Build history of the part. All positions in model axes, mm. A direction names the side the tool comes from. Round coordinates to 2 decimals unless told otherwise and drop trailing zeros. Write each loop counter-clockwise with the first axis right and the second up, starting at its lowest first coordinate (ties: lowest second). Pieces come first, ordered by that corner, then holes. Notation, with made-up numbers: (34, 60.25) -> (80, 60.25) arc R27 cw to (80, 90.25) -> close; hole circle Ø9 at (77, 53.5). An arc over 180 degrees is marked (long way). Return JSON: item names as keys, results as strings.
from build123d import *

# Parameters (mm, degrees)
F0_R     = 6
F0_R_2   = 1.25
F3_DEPTH = 12
F4_DEPTH = 12


with BuildPart() as f2:
    # F2: sweep along a path in F1
    with BuildLine(Plane.XZ) as f2_path:
        Line((0, 0), (0, 5))
        ThreePointArc((0, 5), (4.3933982822, 15.6066017178), (15, 20))
        Line((15, 20), (54.5, 20))
        ThreePointArc((54.5, 20), (65.1066017178, 15.6066017178), (69.5, 5))
        Line((69.5, 5), (69.5, 0))
    # F0 (on Top) → F2 (sweep)
    with BuildSketch(Plane.XY):
        Circle(F0_R)
        Circle(F0_R_2, mode=Mode.SUBTRACT)
        Circle(F0_R_2)
    sweep(path=f2_path.line)

    # F0 (on Top) → F3 (cut)
    with BuildSketch(Plane.XY):
        Circle(F0_R_2)
    extrude(amount=F3_DEPTH, mode=Mode.SUBTRACT)

    # F0 (on Top) → F4 (cut)
    with BuildSketch(Plane.XY):
        with BuildLine():
            ThreePointArc((70.75, 0), (69.5, 1.25), (68.25, 0))
            ThreePointArc((68.25, 0), (69.5, -1.25), (70.75, 0))
        make_face()
    extrude(amount=F4_DEPTH, mode=Mode.SUBTRACT)


solid = f2.part
Q1. Wall check: L1, parallel to Y at x = 0, z = 8.5; L2, parallel to X at y = 0.5, z = 11.5; L3, parallel to X at y = 3.5, z = 3. Give the ranges that are in metal, low to high.
Verdict:
{"L1": "y = -5.99 to -1.25, 1.25 to 5.99", "L2": "x = -4.95 to -1.15, 1.15 to 8.74, 60.76 to 68.35, 70.65 to 74.45", "L3": "x = -4.87 to 4.87, 64.63 to 74.37"}
Q2. Saw through at D-D on y = 4. List the corners of the cut face in (x, z).
Verdict:
{"outline": "(-4.47, 0) -> (4.47, 0) -> (4.47, 5) arc R10.53 cw to (15, 15.53) -> (54.5, 15.53) arc R10.53 cw to (65.03, 5) -> (65.03, 0) -> (73.97, 0) -> (73.97, 5) arc R19.47 ccw to (54.5, 24.47) -> (15, 24.47) arc R19.47 ccw to (-4.47, 5) -> close"}
Q3. Two-plate mould, pull along X, no slides. Class faces 1 (the flat face through (-0.1, 1.4, 0)), 2 (the cylindrical face through (35.03, -3.65, 24.76)): +X half, -X half, draft (parallel to the pull), parting line (faces both ways), or undercut.
Verdict:
{"face 1": "draft", "face 2": "undercut"}
Q4. Saw through at C-C on x = 30. List the corners of the cut face in (y, z), then the cut area to 3 significant figures.
Verdict:
{"outline": "circle Ø12 at (0, 20)", "area": "113 mm²"}
Q5. Saw through at B-B on z = 3.5. List the corners of the cut face in (x, y).
Verdict:
{"outline": "circle Ø12 at (0, 0); circle Ø12 at (69.5, 0); hole circle Ø2.5 at (0, 0); hole circle Ø2.5 at (69.5, 0)"}
Q6. Pin check, flat tips, straight feed: pin 1 Ø12 at (x, z) = (57.5, 17) entering from +Y; pin 2 Ø3 at (x, y) = (50, 4.5) entering from +Z; pin 3 Ø4 at (x, y) = (63.5, 0.5) entering from +Z; pin 4 Ø1.5 at (x, y) = (69.5, 0) entering from +Z. Stop position of each tip, or through.
Verdict:
{"pin 1": "stops at y = 6", "pin 2": "stops at z = 25.2", "pin 3": "stops at z = 24.79", "pin 4": "stops at z = 20.43"}
Q7. Saw through at A-A on y = 0. List the corners of the cut face in (x, z), then the cut area to 3 significant figures.
Verdict:
{"outline": "(-6, 0) -> (-1.25, 0) -> (-1.25, 12) -> (1.25, 12) -> (1.25, 0) -> (6, 0) -> (6, 5) arc R9 cw to (15, 14) -> (54.5, 14) arc R9 cw to (63.5, 5) -> (63.5, 0) -> (68.25, 0) -> (68.25, 12) -> (70.75, 12) -> (70.75, 0) -> (75.5, 0) -> (75.5, 5) arc R21 ccw to (54.5, 26) -> (15, 26) arc R21 ccw to (-6, 5) -> close", "area": "1,100 mm²"}
Q8. 3-axis set-ups, long thin cutter, end or side, ignore diameter. For faces 3 (the flat face through (68, 0, 0)), 4 (the flat face through (69, 0, 12)): which of +Z, -Z, +X, -X, +Y, -Y reach the whole face in a straight line?
Verdict:
{"face 3": "-Z, +X, -X, +Y, -Y", "face 4": "-Z"}
